Verification items for this drawing (mm, ordinates from the low corner). A direction names the side the tool comes from. Coordinates: 2 decimals unless noted, no trailing zeros. Order: outer loops, then holes, each group sorted by start corner. A loop starts at its lowest first (then second) coordinate and runs counter-clockwise, first axis right, second up.
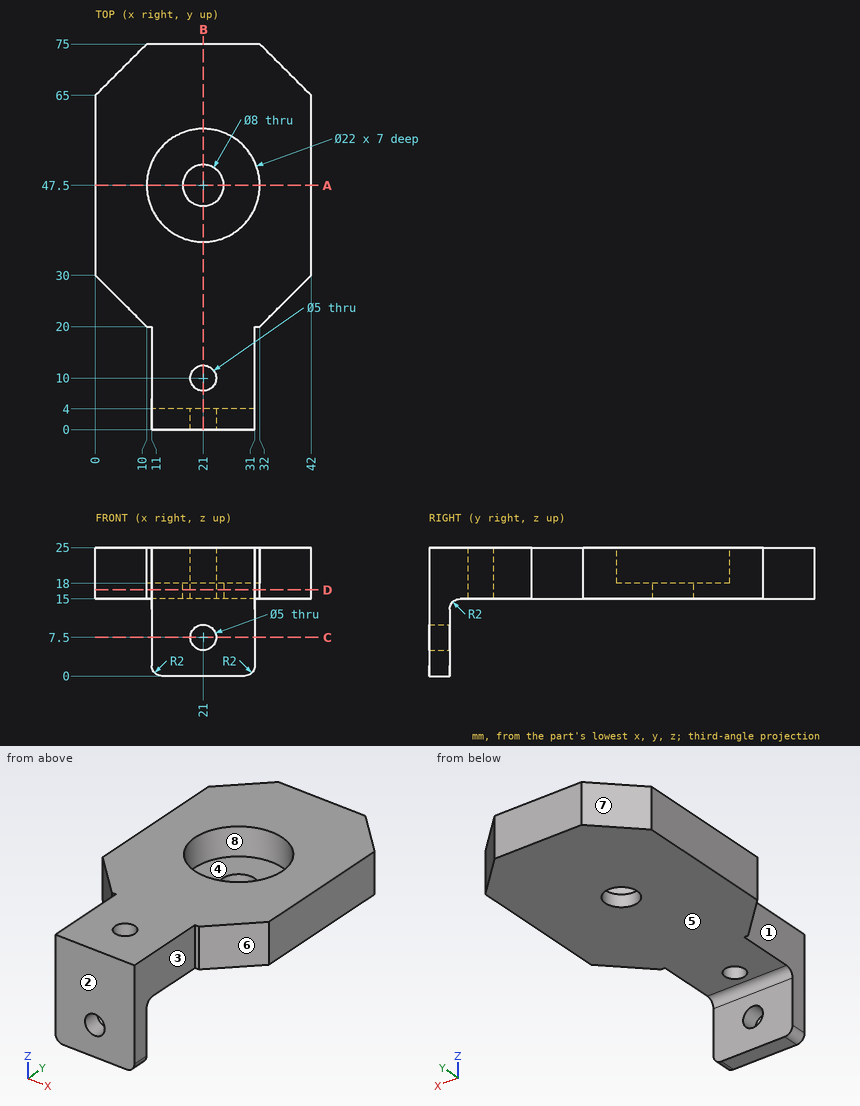
(1) Go/stop test with flat-tipped pins: P1, Ø4, axis at x = 21, y = 10, coming from the +Z side; P2, Ø6, axis at y = 5.5, z = 12.5, coming from the +X side; P3, Ø4, axis at x = 23, y = 41.5, coming from the -Z side; P4, Ø4, axis at x = 22.5, z = 9, coming from the +Y side. Record where each tip stops, or that it passes through.
Filled in:
P1: passes through
P2: stops at x = 31
P3: stops at z = 15
P4: stops at y = 4
(2) Release check for a two-part mould opening along X. For the marked faces 6, 7 and 8 record: +X half, -X half, draft (parallel to the pull), parting line (faces both ways), or undercut.
Filled in:
face 6: +X half
face 7: -X half
face 8: undercut
(3) Cross-section at B-B (x = 21). Enter the section's corners in (y, z).
Filled in:
outline: (0, 0) - (4, 0) - (4, 5) - (0, 5) - close; (0, 10) - (4, 10) - (4, 13) arc R2 cw to (6, 15) - (7.5, 15) - (7.5, 25) - (0, 25) - close; (12.5, 15) - (43.5, 15) - (43.5, 18) - (36.5, 18) - (36.5, 25) - (12.5, 25) - close; (51.5, 15) - (75, 15) - (75, 25) - (58.5, 25) - (58.5, 18) - (51.5, 18) - close
(4) Cross-section at D-D (z = 16.75). Enter the section's corners in (x, y), and give its area (3 significant figures).
Filled in:
outline: (0, 30) - (10, 20) - (11, 20) - (11, 0) - (31, 0) - (31, 20) - (32, 20) - (42, 30) - (42, 65) - (32, 75) - (10, 75) - (0, 65) - close; hole circle Ø8 at (21, 47.5); hole circle Ø5 at (21, 10)
area: 2,440 mm2
(5) Cross-section at C-C (z = 7.5). Enter the section's corners in (x, y).
Filled in:
outline: (11, 0) - (18.5, 0) - (18.5, 4) - (11, 4) - close; (23.5, 0) - (31, 0) - (31, 4) - (23.5, 4) - close
(6) Thickness scan on probe 1 along Y at (x, z) = (21, 17.5); probe 2 along Z at (x, y) = (21, 1.65); probe 3 along Y at (x, z) = (21, 21). Record the ranges inside material, lowest first.
Filled in:
probe 1: y = 0 to 7.5, 12.5 to 43.5, 51.5 to 75
probe 2: z = 0 to 5, 10 to 25
probe 3: y = 0 to 7.5, 12.5 to 36.5, 58.5 to 75
(7) Cross-section at A-A (y = 47.5). Enter the section's corners in (x, z).
Filled in:
outline: (0, 15) - (17, 15) - (17, 18) - (10, 18) - (10, 25) - (0, 25) - close; (25, 15) - (42, 15) - (42, 25) - (32, 25) - (32, 18) - (25, 18) - close
(8) Tool access check on the marked faces 1, 2, 3, 4 and 5. Record the directions out of +Z, -Z, +X, -X, +Y, -Y that give a thin tool (end or side, any length) a straight path to the whole face; none if there is none.
Filled in:
face 1: +Z, -Z, -X, -Y
face 2: +Z, -Z, +X, -X, -Y
face 3: +Z, -Z, +X, -Y
face 4: +Z
face 5: -Z, +X, -X, +Y
